Source: three-view drawing plus pictorial views. Frame: mm from the lowest corner of the part. A direction names the side the tool comes from. Coordinates: 2 decimals unless noted, no trailing zeros. Write each loop counter-clockwise with the first axis right and the second up, starting at its lowest first coordinate (ties: lowest second). Pieces come first, ordered by that corner, then holes. Notation, with made-up numbers: (-28, 61) -> (10, 61) arc R10 cw to (10, 75) -> close; hole circle Ø1 at (32.25, -36.5). An arc over 180 degrees is marked (long way). One line per item, written item: value. Start each with the question number.
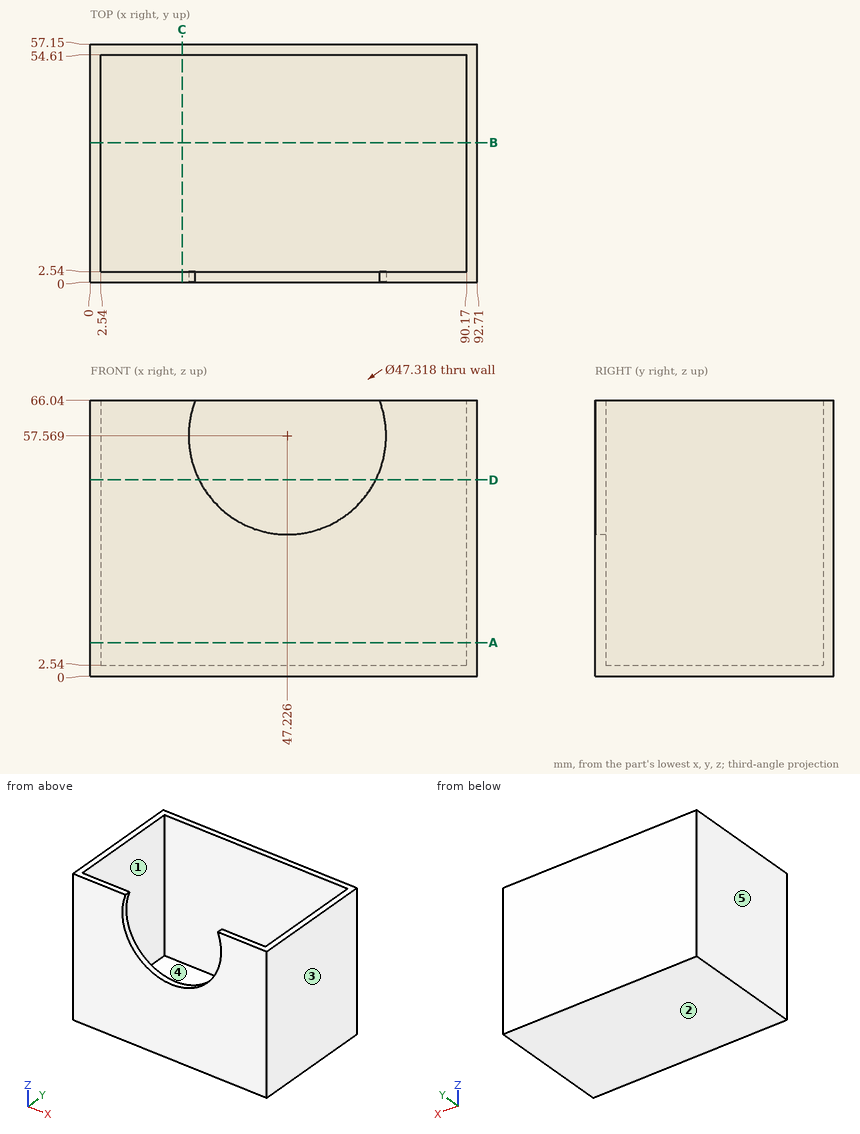
Q1. Cut plane C-C on x = 22. Output: boundary loops of the cut face in (y, z).
Q2. Cut plane A-A on z = 8. Output: boundary loops of the cut face in (x, y).
Q3. Cut plane D-D on z = 47. Output: boundary loops of the cut face in (x, y), and give its area (3 significant figures).
Q4. Draft query along X for the marked faces 1, 2 and 3. Return one class per face: pulls with the +X half, pulls with the -X half, needs draft (parallel to the pull), parting line crosses it, or undercut.
Q5. Line query: L1, parallel to Y at x = 12, z = 46; L2, parallel to X at y = 8, z = 30; L3, parallel to Z at x = 24, y = 7.5. Output: solid intervals per line, ascending. Write a range as from..to.
Q6. Cut plane B-B on y = 33.5. Output: boundary loops of the cut face in (x, z).
Q7. First-contact query: P1, Ø3, axis at x = 24.5, y = 18, coming from the +Z side; P2, Ø3, axis at x = 47, z = 21, coming from the -Y side. Flat tips, straight axial feed; report the tip coordinate or a pass-through.
Q8. Access query for the marked faces 4 and 5. Directions: +Z, -Z, +X, -X, +Y, -Y. A direction counts if a zero-diameter tool reaches every point of the face in a straight line with its end or side. Return the directions, or none.
Solution:
1. outline: (0, 0) -> (57.15, 0) -> (57.15, 66.04) -> (54.61, 66.04) -> (54.61, 2.54) -> (2.54, 2.54) -> (2.54, 66.04) -> (0, 66.04) -> close
2. outline: (0, 0) -> (92.71, 0) -> (92.71, 57.15) -> (0, 57.15) -> close; hole (2.54, 2.54) -> (90.17, 2.54) -> (90.17, 54.61) -> (2.54, 54.61) -> close
3. outline: (0, 0) -> (26.06, 0) -> (26.06, 2.54) -> (2.54, 2.54) -> (2.54, 54.61) -> (90.17, 54.61) -> (90.17, 2.54) -> (68.39, 2.54) -> (68.39, 0) -> (92.71, 0) -> (92.71, 57.15) -> (0, 57.15) -> close
3. area: 628 mm²
4. face 1: undercut
4. face 2: needs draft
4. face 3: pulls with the +X half
5. L1: 0..2.54, 54.61..57.15
5. L2: 0..2.54, 90.17..92.71
5. L3: 0..2.54
6. outline: (0, 0) -> (92.71, 0) -> (92.71, 66.04) -> (90.17, 66.04) -> (90.17, 2.54) -> (2.54, 2.54) -> (2.54, 66.04) -> (0, 66.04) -> close
7. P1: z = 2.54
7. P2: y = 0
8. face 4: +Z
8. face 5: +Z, -Z, -X, +Y, -Y
